```python
from build123d import *

# Parameters (mm, degrees)
SKETCH3_W           = 100
SKETCH3_H           = 80
BOSS_EXTRUDE1_DEPTH = 90
CUT_EXTRUDE1_DEPTH  = 90
CUT_EXTRUDE2_DEPTH  = 90
CUT_EXTRUDE3_DEPTH  = 90
SKETCH8_W           = 40
SKETCH8_H           = 60
CUT_EXTRUDE4_DEPTH  = 60
SKETCH9_W           = 30
SKETCH9_H           = 30
CUT_EXTRUDE5_DEPTH  = 60
SKETCH10_W          = 10
SKETCH10_H          = 10
CUT_EXTRUDE6_DEPTH  = 60
SKETCH11_W          = 40
SKETCH11_H          = 60
BOSS_EXTRUDE2_DEPTH = 20
SKETCH12_W          = 40
SKETCH12_H          = 20
BOSS_EXTRUDE3_DEPTH = 40
SKETCH13_W          = 30
SKETCH13_H          = 10
CUT_EXTRUDE7_DEPTH  = 40
CUT_EXTRUDE8_DEPTH  = 40
CUT_EXTRUDE9_DEPTH  = 20
SKETCH17_W          = 20
SKETCH17_H          = 20
CUT_EXTRUDE10_DEPTH = 84
CUT_EXTRUDE12_DEPTH = 20
CUT_EXTRUDE15_DEPTH = 10
CUT_EXTRUDE17_DEPTH = 77
CUT_EXTRUDE19_DEPTH = 77
CUT_EXTRUDE20_DEPTH = 77
CUT_EXTRUDE21_DEPTH = 77


with BuildPart() as part:
    # Sketch3 → Boss-Extrude1 (new body)
    with BuildSketch(Plane.XY):
        with Locations((50, 40)):
            Rectangle(SKETCH3_W, SKETCH3_H)
    extrude(amount=-BOSS_EXTRUDE1_DEPTH)

    # Sketch4 → Cut-Extrude1 (cut)
    with BuildSketch(Plane.XY):
        Polygon((20, 80), (20, 70), (60, 70), (80, 50), (80, 30), (100, 30), (100, 80), align=None)
    extrude(amount=-CUT_EXTRUDE1_DEPTH, mode=Mode.SUBTRACT)

    # Sketch5 → Cut-Extrude2 (cut)
    with BuildSketch(Plane(origin=(0, 0, 0), x_dir=(-1, 0, 0), z_dir=(0, -1, 0))):
        Polygon((-70, 0), (-100, 30), (-100, 0), align=None)
    extrude(amount=-CUT_EXTRUDE2_DEPTH, mode=Mode.SUBTRACT)

    # Sketch7 → Cut-Extrude3 (cut)
    with BuildSketch(Plane.ZY):
        Polygon((-40, 80), (0, 40), (0, 80), align=None)
    extrude(amount=-CUT_EXTRUDE3_DEPTH, mode=Mode.SUBTRACT)

    # Sketch8 → Cut-Extrude4 (cut)
    with BuildSketch(Plane(origin=(0, 70, 0), x_dir=(1, 0, 0), z_dir=(0, 1, 0))):
        with Locations((40, 60)):
            Rectangle(SKETCH8_W, SKETCH8_H)
    extrude(amount=-CUT_EXTRUDE4_DEPTH, mode=Mode.SUBTRACT)

    # Sketch9 → Cut-Extrude5 (cut)
    with BuildSketch(Plane(origin=(0, 0, -30), x_dir=(-1, 0, 0), z_dir=(0, 0, -1))):
        with Locations((-45, 55)):
            Rectangle(SKETCH9_W, SKETCH9_H)
    extrude(amount=-CUT_EXTRUDE5_DEPTH, mode=Mode.SUBTRACT)

    # Sketch10 → Cut-Extrude6 (cut)
    with BuildSketch(Plane(origin=(0, 0, -30), x_dir=(-1, 0, 0), z_dir=(0, 0, -1))):
        with Locations((-25, 65)):
            Rectangle(SKETCH10_W, SKETCH10_H)
    extrude(amount=-CUT_EXTRUDE6_DEPTH, mode=Mode.SUBTRACT)

    # Sketch11 → Boss-Extrude2 (add)
    with BuildSketch(Plane(origin=(0, 10, 0), x_dir=(1, 0, 0), z_dir=(0, 1, 0))):
        with Locations((40, 60)):
            Rectangle(SKETCH11_W, SKETCH11_H)
    extrude(amount=BOSS_EXTRUDE2_DEPTH)

    # Sketch12 → Boss-Extrude3 (add)
    with BuildSketch(Plane(origin=(0, 30, 0), x_dir=(1, 0, 0), z_dir=(0, 1, 0))):
        with Locations((40, 80)):
            Rectangle(SKETCH12_W, SKETCH12_H)
    extrude(amount=BOSS_EXTRUDE3_DEPTH)

    # Sketch13 → Cut-Extrude7 (cut)
    with BuildSketch(Plane(origin=(0, 0, -30), x_dir=(-1, 0, 0), z_dir=(0, 0, -1))):
        with Locations((-45, 35)):
            Rectangle(SKETCH13_W, SKETCH13_H)
    extrude(amount=-CUT_EXTRUDE7_DEPTH, mode=Mode.SUBTRACT)

    # Sketch15 → Cut-Extrude8 (cut)
    with BuildSketch(Plane.ZY.offset(-60)):
        Polygon((-70, 70), (-70, 30), (0, 30), (0, 40), (-30, 70), align=None)
    extrude(amount=-CUT_EXTRUDE8_DEPTH, mode=Mode.SUBTRACT)

    # Sketch16 → Cut-Extrude9 (cut)
    with BuildSketch(Plane(origin=(0, 30, 0), x_dir=(1, 0, 0), z_dir=(0, 1, 0))):
        Polygon((100, 80), (80, 60), (40, 60), (40, 20), (80, 20), (100, 40), align=None)
    extrude(amount=-CUT_EXTRUDE9_DEPTH, mode=Mode.SUBTRACT)

    # Sketch17 → Cut-Extrude10 (cut)
    with BuildSketch(Plane.XY.offset(-50)):
        with Locations((90, 20)):
            Rectangle(SKETCH17_W, SKETCH17_H)
    extrude(amount=CUT_EXTRUDE10_DEPTH, mode=Mode.SUBTRACT)

    # Sketch19 → Cut-Extrude12 (cut)
    with BuildSketch(Plane.XY.offset(-10)):
        Polygon((80, 10), (60, 30), (80, 30), align=None)
    extrude(amount=CUT_EXTRUDE12_DEPTH, mode=Mode.SUBTRACT)

    # Sketch22 → Cut-Extrude15 (cut)
    with BuildSketch(Plane.XY.offset(-10)):
        Polygon((60, 30), (80, 30), (80, 10), align=None)
    extrude(amount=-CUT_EXTRUDE15_DEPTH, mode=Mode.SUBTRACT)

    # Sketch24 → Cut-Extrude17 (cut)
    with BuildSketch(Plane(origin=(23.333333333, 23.333333333, 23.333333333), x_dir=(0.40824829, 0.40824829, -0.816496581), z_dir=(0.577350269, 0.577350269, 0.577350269))):
        Polygon((53.07227776, -21.213203436), (28.577380332, -7.071067812), (28.577380332, -49.497474683), (53.07227776, -49.497474683), align=None)
    extrude(amount=CUT_EXTRUDE17_DEPTH, mode=Mode.SUBTRACT)

    # Sketch26 → Cut-Extrude19 (cut)
    with BuildSketch(Plane(origin=(35, -35, 0), x_dir=(0, 0, 1), z_dir=(-0.707106781, 0.707106781, 0))):
        Polygon((-20, 63.639610307), (-10, 63.639610307), (0, 49.497474683), align=None)
    extrude(amount=-CUT_EXTRUDE19_DEPTH, mode=Mode.SUBTRACT)

    # Sketch27 → Cut-Extrude20 (cut)
    with BuildSketch(Plane(origin=(45, 45, 0), x_dir=(0, 0, 1), z_dir=(-0.707106781, -0.707106781, 0))):
        Polygon((-20, -49.497474683), (-10, -49.497474683), (-20, -63.639610307), align=None)
    extrude(amount=-CUT_EXTRUDE20_DEPTH, mode=Mode.SUBTRACT)

    # Sketch30 → Cut-Extrude21 (cut)
    with BuildSketch(Plane(origin=(23.333333333, 23.333333333, 23.333333333), x_dir=(-0.816496581, 0.40824829, 0.40824829), z_dir=(-0.577350269, -0.577350269, -0.577350269))):
        Polygon((-69.402209379, 21.213203436), (-93.897106807, 35.355339059), (-93.897106807, 21.213203436), (-81.649658093, 14.142135624), align=None)
    extrude(amount=-CUT_EXTRUDE21_DEPTH, mode=Mode.SUBTRACT)


solid = part.part
```
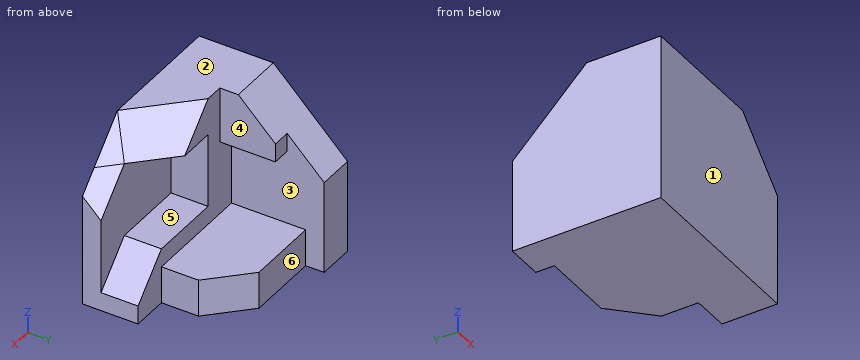
Verification items for the finished model (mm, model axes). Face numbers are marked on the shaded views. A direction names the side the tool comes from. Give positions to 0.01 mm unless a question says otherwise; leave off trailing zeros. Loops run counter-clockwise (first coordinate to the right, second up) from the corner with the lowest first, then second, coordinate; pieces in that order, holes last.
1. Section check C-C, the plane z = -78. Enter the section's corners in (x, y), then the cut area to 3 significant figures.
2. Mould release check, pull along Z, two halves, no side actions. Record for the marked faces 1, 2 and 3: released by +Z, released by -Z, zero draft, split by the parting line, or undercut.
3. Thickness scan on line 1 (Z direction, x = 44.5, y = 11.5); line 2 (Y direction, x = 81, z = -34); line 3 (Y direction, x = 86, z = -74.5). Record the ranges inside material, lowest first.
4. Section check D-D, the plane x = 23. Enter the section's corners in (y, z), then the cut area to 3 significant figures.
5. Set-up check for the marked faces 4, 5 and 6: record each of +Z, -Z, +X, -X, +Y, -Y from which the full face is reachable in a straight line by a thin tool's end or side.
6. Section check B-B, the plane x = 54.5. Enter the section's corners in (y, z).
7. Section check A-A, the plane y = 20. Enter the section's corners in (x, z), then the cut area to 3 significant figures.
8. Go/stop test with flat-tipped pins: pin 1 Ø6 at (x, y) = (56.5, 71.5) entering from -Z; pin 2 Ø10 at (y, z) = (38.5, -77.5) entering from +X; pin 3 Ø12 at (x, z) = (37, -38) entering from +Y; pin 4 Ø10 at (x, z) = (38.5, -82.5) entering from +Y. Record where each tip stops, or that it passes through.
Geometry says:
1. outline: (0, 0) - (100, 0) - (100, 10) - (98, 10) - (98, 30) - (80, 30) - (80, 50) - (60, 70) - (20, 70) - (20, 80) - (0, 80) - close
1. area: 6,160 mm2
2. face 1: zero draft
2. face 2: released by +Z
2. face 3: undercut
3. line 1: z = -90 to -60, -20 to 0
3. line 2: y = 0 to 10
3. line 3: y = 0 to 30
4. outline: (0, -90) - (70, -90) - (70, -70) - (30, -70) - (30, -30) - (60, -30) - (60, -20) - (40, 0) - (0, 0) - close
4. area: 4,200 mm2
5. face 4: +Z, +X, +Y
5. face 5: +X, +Y
5. face 6: +Z, -Z, +X, +Y
6. outline: (0, -90) - (70, -90) - (70, -70) - (30, -70) - (30, -60) - (10, -60) - (10, -20) - (30, -20) - (30, -14.5) - (15.5, 0) - (0, 0) - close
7. outline: (0, -90) - (100, -90) - (100, -80) - (80, -60) - (40, -60) - (40, -20) - (70, -20) - (50, 0) - (0, 0) - close
7. area: 5,600 mm2
8. pin 1: stops at z = -90
8. pin 2: stops at x = 80
8. pin 3: stops at y = 30
8. pin 4: stops at y = 70
